Check sheet for the modelled part. Datum: model origin and axes. Units: mm. Give positions to 0.01 mm unless a question says otherwise; leave off trailing zeros. Write each loop counter-clockwise with the first axis right and the second up, starting at its lowest first coordinate (ties: lowest second). Pieces come first, ordered by that corner, then holes. Notation, with made-up numbers: (-22.5, 79) -> (-9.5, 79) arc R27 cw to (-9.5, 107) -> close; hole circle Ø10 at (-24.75, -11). An arc over 180 degrees is marked (long way). Answer as a JSON object with one key per item and string values.
Autodesk Inventor part; units mm, degrees
ref_plane "YZ Plane" through (0, 0, 0) normal (1, 0, 0) x (0, 1, 0)
ref_plane "XZ Plane" through (0, 0, 0) normal (0, 1, 0) x (-1, 0, 0)
ref_plane "XY Plane" through (0, 0, 0) normal (0, 0, 1) x (1, 0, 0)
sketch "Sketch1" plane through (0, 0, 0) normal (0, 0, 1) x (1, 0, 0)
  line L0 (0, 0) -> (-6.8345, 0)
  line L1 (-6.8345, 0) -> (18.5655, 0)
  line L2 (18.5655, 0) -> (18.5655, 50.8)
  line L3 (18.5655, 50.8) -> (-6.8345, 50.8)
  line L4 (-6.8345, 50.8) -> (-6.8345, 0)
  dimension "d0" = 25.4
  dimension "d1" = 50.8
extrude "Extrusion1" add sketch "Sketch1" along normal blind 3.175
sketch "Sketch2" plane through (0, 0, 3.175) normal (0, 0, 1) x (1, 0, 0)
  circle A0 centre (5.8655, 15.875) radius 3.3782
  circle A1 centre (8.6877, 38.1) radius 3.302
  point P0 (0, 0)
extrude "Extrusion2" cut sketch "Sketch2" against normal blind 25.4
sketch "Sketch3" plane through (0, 0, 3.175) normal (0, 0, 1) x (1, 0, 0)
  line L0 (-6.8345, 0) -> (18.5655, 0)
  line L1 (18.5655, 0) -> (18.5655, 50.8)
  line L2 (-6.8345, 50.8) -> (-6.8345, 0)
  line L3 (-6.8345, 0) -> (-6.8345, 6.35)
  line L4 (-6.8345, 6.35) -> (18.5655, 6.35)
  point P0 (0, 0)
  dimension "d6" = 6.35
extrude "Extrusion3" cut sketch "Sketch3" against normal blind 25.4
properties part number "winch mount back support"
1. Mould release check, pull along Y, two halves, no side actions. Record for faces 1 (the face through (6, 29, 3.175)), 2 (the face through (6, 6.35, 2)), 3 (the face through (6, 50.8, 2)), 4 (the face through (7.682, 18.724, 1.61)): released by +Y, released by -Y, zero draft, split by the parting line, or undercut.
Determined:
{"face 1": "zero draft", "face 2": "released by -Y", "face 3": "released by +Y", "face 4": "undercut"}
2. Sectioned sample at B-B, the plane x = 3. Enter the section's corners in (y, z) (3 decimals), plus the area to 3 significant figures.
Determined:
{"outline": "(6.35, 0) -> (14.086, 0) -> (14.086, 3.175) -> (6.35, 3.175) -> close; (17.664, 0) -> (50.8, 0) -> (50.8, 3.175) -> (17.664, 3.175) -> close", "area": "130 mm^2"}
3. Scan lines: L1, parallel to Y at x = 6.5, z = 0.95; L2, parallel to X at y = 38, z = 1.2; L3, parallel to X at y = 15.5, z = 0.25. Record each from-to range of solid material in increasing order. Write a range as [from, to].
Determined:
{"L1": "[6.35, 12.56], [19.19, 35.63], [40.57, 50.8]", "L2": "[-6.83, 5.39], [11.99, 18.57]", "L3": "[-6.83, 2.51], [9.22, 18.57]"}
4. Sectioned sample at C-C, the plane z = 1.75. State how many separate pieces and enclosed holes the cut face has, plus the area to 3 significant figures.
Determined:
{"separate pieces": "1", "enclosed holes": "2", "area": "1,060 mm^2"}
5. Sectioned sample at A-A, the plane y = 38.1. Enter the section's corners in (x, z) (1 decimal).
Determined:
{"outline": "(-6.8, 0) -> (5.4, 0) -> (5.4, 3.2) -> (-6.8, 3.2) -> close; (12, 0) -> (18.6, 0) -> (18.6, 3.2) -> (12, 3.2) -> close"}
